```python
from build123d import *

# Parameters (mm, degrees)
SKETCH1_W            = 61.35
SKETCH1_H            = 86.35
BOSS_EXTRUDE1_DEPTH  = 3.175
SKETCH2_W            = 20
SKETCH2_H            = 3.5
BOSS_EXTRUDE2_DEPTH  = 3.175
CUT_EXTRUDE1_DEPTH   = 3.175
MIRROR2_COPY_1_DEPTH = 3.175


with BuildPart() as part:
    # Sketch1 → Boss-Extrude1 (new body)
    with BuildSketch(Plane(origin=(0, 0, 0), x_dir=(1, 0, 0), z_dir=(0, 1, 0))):
        with Locations((30.675, 43.175)):
            Rectangle(SKETCH1_W, SKETCH1_H)
    extrude(amount=BOSS_EXTRUDE1_DEPTH)

    # Sketch2 → Boss-Extrude2 (add)
    with BuildSketch(Plane.XZ):
        with Locations((33.85, 1.75)):
            Rectangle(SKETCH2_W, SKETCH2_H)
    boss_extrude2 = extrude(amount=-BOSS_EXTRUDE2_DEPTH)

    # Sketch3 → Cut-Extrude1 (cut)
    with BuildSketch(Plane(origin=(0, 3.175, 0), x_dir=(1, 0, 0), z_dir=(0, 1, 0))):
        Polygon((16.35, 0), (16.35, 4), (17.35, 4), (17.35, 7.5), (13.35, 7.5), (13.35, 4), (14.35, 4), (14.35, 0), align=None)
    cut_extrude1 = extrude(amount=-CUT_EXTRUDE1_DEPTH, mode=Mode.SUBTRACT)

    # Mirror1: Cut-Extrude1 across plane
    add(cut_extrude1.mirror(Plane(origin=(33.85, 0, 0), x_dir=(0, 0, 1), z_dir=(1, 0, 0))), mode=Mode.SUBTRACT)

    # Mirror2: Boss-Extrude2, Cut-Extrude1 across plane
    add(boss_extrude2.mirror(Plane.XY.offset(-43.175)))
    add(cut_extrude1.mirror(Plane.XY.offset(-43.175)), mode=Mode.SUBTRACT)

    # Mirror2 copy 1 sketch → Mirror2 copy 1 (cut)
    with BuildSketch(Plane(origin=(67.7, 3.175, -86.35), x_dir=(-1, 0, 0), z_dir=(0, 1, 0))):
        Polygon((16.35, 0), (16.35, 4), (17.35, 4), (17.35, 7.5), (13.35, 7.5), (13.35, 4), (14.35, 4), (14.35, 0), align=None)
    extrude(amount=-MIRROR2_COPY_1_DEPTH, mode=Mode.SUBTRACT)


solid = part.part
```
Can you work these out from the model? Positions are in its coordinate system, mm. A direction names the side the tool comes from. Give positions to 0.01 mm unless a question says otherwise; leave off trailing zeros. Write each loop counter-clockwise with the first axis right and the second up, starting at its lowest first coordinate (ties: lowest second). Pieces come first, ordered by that corner, then holes. Notation, with made-up numbers: (29.25, 45.25) -> (79.25, 45.25) arc R12 cw to (79.25, 65.25) -> close; hole circle Ø2 at (-17, -10). An arc over 180 degrees is marked (long way). Write item = value, one per line.
(1) I'm going to push flat-ended pins straight in: P1, Ø10, axis at x = 20.5, z = -27.5, coming from the -Y side; P2, Ø1, axis at x = 56.5, y = 2.5, coming from the +Z side. Where does each tip first touch, or does it pass through?
Worked out:
P1 = 0
P2 = 0
(2) For faces 5 (the face through (57, 2, 0)), 6 (the face through (7, 2, -86.35)), 7 (the face through (23.85, 2, 2)), 8 (the face through (13.35, 2, -81)), 9 (the face through (51.35, 2, -2)), which set-ups out of +Z, -Z, +X, -X, +Y, -Y let a thin tool reach every point of the face, with its end or its side?
Worked out:
face_5 = +Z, +X, +Y, -Y
face_6 = -Z, -X, +Y, -Y
face_7 = +Z, -X, +Y, -Y
face_8 = +Y, -Y
face_9 = +Z, +Y, -Y
(3) Suppose I cut it at A-A on x = 21. Write out the boundary of the cut face in (y, z) (3 decimals).
Worked out:
outline = (0, -86.35) -> (3.175, -86.35) -> (3.175, 0) -> (0, 0) -> close
(4) Thinking about a two-plate mould opening in X: for faces 1 (the face through (7, 2, 0)), 2 (the face through (43.85, 2, -88)), 3 (the face through (54.35, 2, -6)), 4 (the face through (50.35, 2, -81)), which applies, released by +X, released by -X, zero draft, split by the parting line, or undercut?
Worked out:
face_1 = zero draft
face_2 = released by +X
face_3 = undercut
face_4 = undercut
(5) I need wall thicknesses on probe 1 along Z at (x, y) = (16.5, 1.75); probe 2 along X at (y, z) = (1.7, -5); probe 3 along Z at (x, y) = (19, 2.2). Which ranges of each line are inside material? Lowest first, please. Write a range as from..to.
Worked out:
probe_1 = -86.35..-82.35, -78.85..-7.5, -4..0
probe_2 = 0..13.35, 17.35..50.35, 54.35..61.35
probe_3 = -86.35..0
